Input: part model. Units: mm. Frame: model coordinates. Face numbers are marked on the shaded views. Give positions to 0.01 mm unless a question says otherwise; leave off trailing zeros. Loops run counter-clockwise (first coordinate to the right, second up) from the corner with the lowest first, then second, coordinate; pieces in that order, holes last.
from build123d import *

# Parameters (mm, degrees)
F1_DEPTH = 8.001
F3_DEPTH = 3.937
F5_DEPTH = 27.94
F7_DEPTH = 62.865
F8_R     = 2.159
F9_DEPTH = 25.4
F10_SIZE = 2.032
F11_R    = 0.762


with BuildPart() as f1:
    # F0 (on Top) → F1 (new body)
    with BuildSketch(Plane.XY):
        with BuildLine():
            Line((31.4325, 61.9125), (-31.4325, 61.9125))
            ThreePointArc((-31.4325, 61.9125), (-52.9851146906, 52.9851146906), (-61.9125, 31.4325))
            Line((-61.9125, 31.4325), (-61.9125, -31.4325))
            ThreePointArc((-61.9125, -31.4325), (-52.9851146906, -52.9851146906), (-31.4325, -61.9125))
            Line((-31.4325, -61.9125), (31.4325, -61.9125))
            ThreePointArc((31.4325, -61.9125), (52.9851146906, -52.9851146906), (61.9125, -31.4325))
            Line((61.9125, -31.4325), (61.9125, 31.4325))
            ThreePointArc((61.9125, 31.4325), (52.9851146906, 52.9851146906), (31.4325, 61.9125))
        make_face()
    extrude(amount=F1_DEPTH)

    # F2 (on face) → F3 (cut)
    with BuildSketch(Plane.XY.offset(8.001)):
        with BuildLine():
            Line((31.4325, 60.325), (-31.4325, 60.325))
            ThreePointArc((-31.4325, 60.325), (-51.8625826754, 51.8625826754), (-60.325, 31.4325))
            Line((-60.325, 31.4325), (-60.325, -31.4325))
            ThreePointArc((-60.325, -31.4325), (-51.8625826754, -51.8625826754), (-31.4325, -60.325))
            Line((-31.4325, -60.325), (31.4325, -60.325))
            ThreePointArc((31.4325, -60.325), (51.8625826754, -51.8625826754), (60.325, -31.4325))
            Line((60.325, -31.4325), (60.325, 31.4325))
            ThreePointArc((60.325, 31.4325), (51.8625826754, 51.8625826754), (31.4325, 60.325))
        make_face()
    extrude(amount=-F3_DEPTH, mode=Mode.SUBTRACT)

    # F4 (on face) → F5 (join)
    with BuildSketch(Plane.XY.offset(8.001)):
        with BuildLine():
            Line((61.9125, 31.4325), (60.325, 31.4325))
            Line((60.325, 31.4325), (60.325, -31.4325))
            ThreePointArc((60.325, -31.4325), (51.8625826754, -51.8625826754), (31.4325, -60.325))
            Line((31.4325, -60.325), (31.4325, -61.9125))
            ThreePointArc((31.4325, -61.9125), (52.9851146906, -52.9851146906), (61.9125, -31.4325))
            Line((61.9125, -31.4325), (61.9125, 31.4325))
        make_face()
        with BuildLine():
            Line((-60.325, -31.4325), (-60.325, 31.4325))
            Line((-60.325, 31.4325), (-61.9125, 31.4325))
            Line((-61.9125, 31.4325), (-61.9125, -31.4325))
            ThreePointArc((-61.9125, -31.4325), (-52.9851146906, -52.9851146906), (-31.4325, -61.9125))
            Line((-31.4325, -61.9125), (-31.4325, -60.325))
            ThreePointArc((-31.4325, -60.325), (-51.8625826754, -51.8625826754), (-60.325, -31.4325))
        make_face()
    extrude(amount=F5_DEPTH)

    # F6 (on face) → F7 (join, through all)
    with BuildSketch(Plane(origin=(0, 31.4325, 0), x_dir=(-1, 0, 0), z_dir=(0, 1, 0))):
        Polygon((-56.8325, 35.941), (-60.325, 35.941), (-60.325, 32.4485), align=None)
        Polygon((60.325, 32.4485), (60.325, 35.941), (56.8325, 35.941), align=None)
    extrude(amount=-F7_DEPTH)

    # F8 (on face) → F9 (cut)
    with BuildSketch(Plane(origin=(0, 0, 0), x_dir=(1, 0, 0), z_dir=(0, 0, -1))):
        with Locations((-31.4325, 31.4325)):
            Circle(F8_R)
        with Locations((31.4325, 31.4325)):
            Circle(F8_R)
        with Locations((31.4325, -31.4325)):
            Circle(F8_R)
        with Locations((-31.4325, -31.4325)):
            Circle(F8_R)
    extrude(amount=-F9_DEPTH, mode=Mode.SUBTRACT)

    # F10
    f10_edges = [f1.edges().sort_by_distance(p)[0] for p in [
        (29.2735, -31.4325, 4.064),
        (-33.5915, -31.4325, 4.064),
        (-33.5915, 31.4325, 4.064),
        (29.2735, 31.4325, 4.064),
    ]]
    chamfer(f10_edges, length=F10_SIZE)

    # F11
    f11_edges = [f1.edges().sort_by_distance(p)[0] for p in [
        (-52.985115, 52.985115, 0),
    ]]
    fillet(f11_edges, radius=F11_R)


solid = f1.part
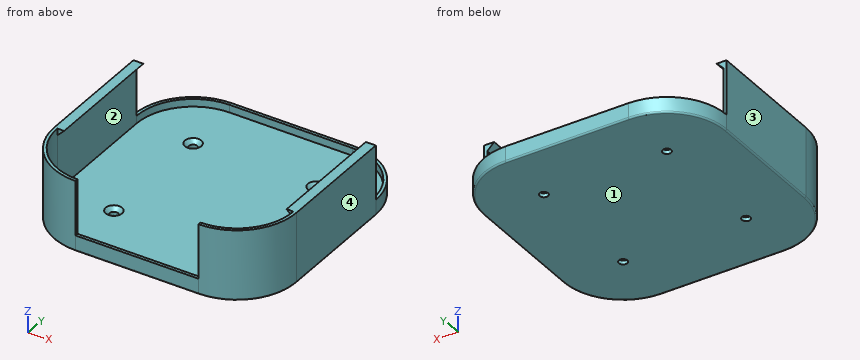
(1) Mould query, pull axis X, two halves, no side actions, for the marked faces 1, 2, 3 and 4. Classes: +X half, -X half, draft (parallel to the pull), parting line (faces both ways), or undercut.
Values follow:
face 1: draft
face 2: undercut
face 3: -X half
face 4: +X half
(2) Ray query, probe 1 along X at (y, z) = (-34.5, 4); probe 2 along X at (y, z) = (-7.5, 30) (1 decimal). Return the intervals inside material, ascending.
Values follow:
probe 1: x = -61.76 to -34.19, -28.67 to 28.67, 34.19 to 61.76
probe 2: x = -61.9 to -60.3, 60.3 to 61.9
(3) Cut plane C-C (y = -3.5). Return the cut outline in (x, z) (1 decimal), and give its area (3 significant figures).
Values follow:
outline: (-61.9, 0.8) arc R0.8 ccw to (-61.2, 0) - (61.2, 0) arc R0.8 ccw to (61.9, 0.8) - (61.9, 35.9) - (56.8, 35.9) - (60.3, 32.4) - (60.3, 4.1) - (-60.3, 4.1) - (-60.3, 32.4) - (-56.8, 35.9) - (-61.9, 35.9) - close
area: 616 mm2
(4) Pin query (flat end, axial travel): pin 1 Ø1 at (x, y) = (27, 22.5) entering from -Z; pin 2 Ø1 at (x, z) = (45, 4) entering from +Y; pin 3 Ø2.5 at (x, z) = (-60, 24) entering from +Y; pin 4 Ø5.5 at (x, y) = (31.43, -31.43) entering from +Z. Return the tip coordinate at first contact, or that it passes through.
Values follow:
pin 1: stops at z = 0
pin 2: stops at y = 58.97
pin 3: stops at y = 31.43
pin 4: stops at z = 2.63
(5) Cut plane A-A (z = 15.5). Return the cut outline in (x, y) (1 decimal), and give its area (3 significant figures).
Values follow:
outline: (-61.9, -31.4) arc R30.5 ccw to (-31.4, -61.9) - (-31.4, -60.3) arc R28.9 cw to (-60.3, -31.4) - (-60.3, 31.4) - (-61.9, 31.4) - close; (31.4, -61.9) arc R30.5 ccw to (61.9, -31.4) - (61.9, 31.4) - (60.3, 31.4) - (60.3, -31.4) arc R28.9 cw to (31.4, -60.3) - close
area: 348 mm2
(6) Cut plane B-B (x = 14). Return the cut outline in (y, z) (1 decimal).
Values follow:
outline: (-61.9, 0.8) arc R0.8 ccw to (-61.2, 0) - (61.2, 0) arc R0.8 ccw to (61.9, 0.8) - (61.9, 8) - (60.3, 8) - (60.3, 4.1) - (-60.3, 4.1) - (-60.3, 8) - (-61.9, 8) - close
